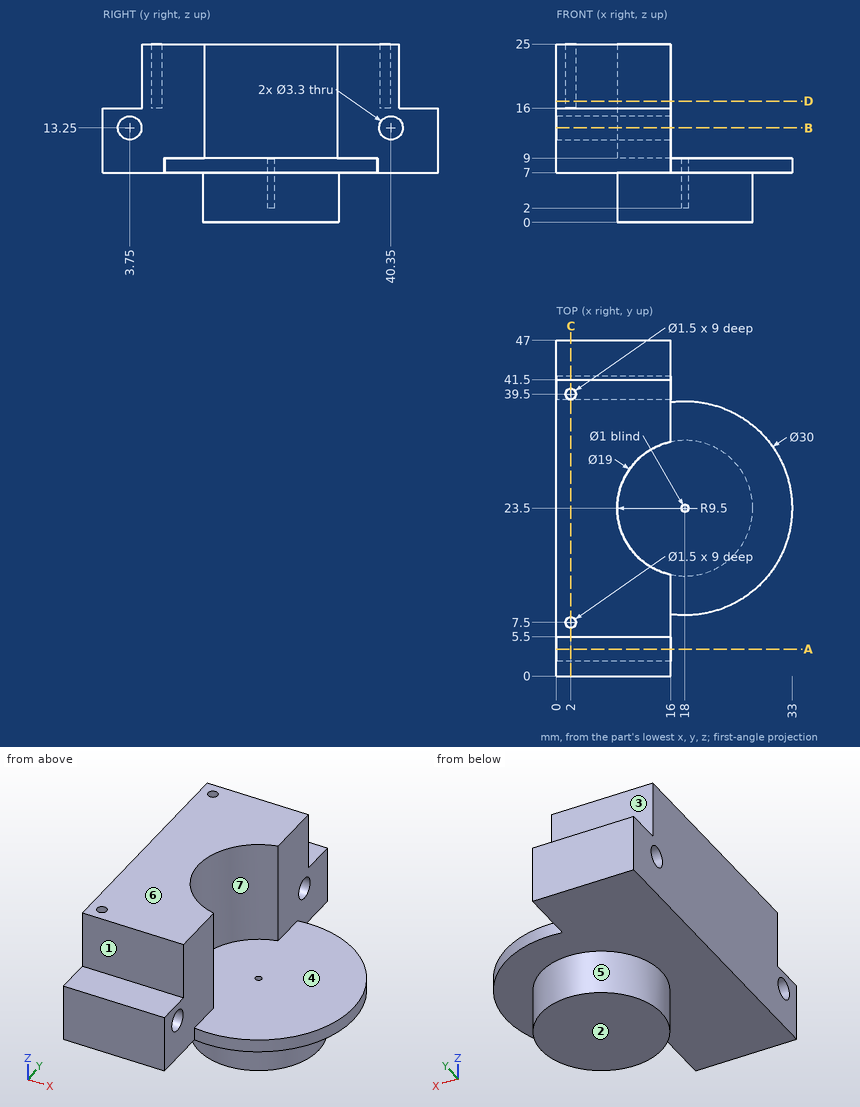
Part print with two shaded views. Sizes in mm from the minimum x, y, z corner. A direction names the side the tool comes from. Give positions to 0.01 mm unless a question says otherwise; leave off trailing zeros. Order: outer loops, then holes, each group sorted by start corner. A loop starts at its lowest first (then second) coordinate and runs counter-clockwise, first axis right, second up. Notation, with made-up numbers: M 12,18 L 46,18 A23 ccw 46,28 Z; hole C 71,-20 d6. An arc over 180 degrees is marked long. Use one line per item in the form item = value.
1) Saw through at A-A (y = 3.75). Give the cut face in (x, z), plus the area to 3 significant figures.
Calculated:
outline = M 0,7 L 16,7 L 16,11.6 L 0,11.6 Z; M 0,14.9 L 16,14.9 L 16,16 L 0,16 Z
area = 91.2 mm2
2) Saw through at D-D (z = 17). Give the cut face in (x, y), plus the area to 3 significant figures.
Calculated:
outline = M 0,5.5 L 16,5.5 L 16,14.21 A9.5 cw 16,32.79 L 16,41.5 L 0,41.5 Z; hole C 2,7.5 d1.5; hole C 2,39.5 d1.5
area = 468 mm2
3) Saw through at C-C (x = 2). Give the cut face in (y, z).
Calculated:
outline = M 0,7 L 47,7 L 47,16 L 41.5,16 L 41.5,25 L 40.25,25 L 40.25,16 L 38.75,16 L 38.75,25 L 8.25,25 L 8.25,16 L 6.75,16 L 6.75,25 L 5.5,25 L 5.5,16 L 0,16 Z; hole C 3.75,13.25 d3.3; hole C 40.35,13.25 d3.3
4) Tool access for the marked faces 1, 2, 3 and 4: list every direction of +Z, -Z, +X, -X, +Y, -Y with a clear straight run to the whole face (end or side of a thin tool).
Calculated:
face_1 = +Z, +X, -X, -Y
face_2 = -Z, +X, -X, +Y, -Y
face_3 = +Z, +X, -X, +Y
face_4 = +Z, +X
5) Probe probe 1 along Z at (x, y) = (10, 40.5); probe 2 along Y at (x, z) = (2, 19.75); probe 3 along Z at (x, y) = (27.5, 12). List the from-to ranges inside material, lowest first.
Calculated:
probe_1 = 7 to 11.61, 14.89 to 25
probe_2 = 5.5 to 6.75, 8.25 to 38.75, 40.25 to 41.5
probe_3 = 7 to 9
6) Saw through at B-B (z = 13.25). Give the cut face in (x, y).
Calculated:
outline = M 0,0 L 16,0 L 16,2.1 L 0,2.1 Z; M 0,5.4 L 16,5.4 L 16,14.21 A9.5 cw 16,32.79 L 16,38.7 L 0,38.7 Z; M 0,42 L 16,42 L 16,47 L 0,47 Z
7) Two-plate mould, pull along Y, no slides. Class the marked faces 5, 6 and 7: released by +Y, released by -Y, zero draft, split by the parting line, or undercut.
Calculated:
face_5 = split by the parting line
face_6 = zero draft
face_7 = undercut
8) Drop flat-ended pins along their axis: pin 1 (7 mm diameter, centred on y = 9, z = 19.5, fed in from +X); pin 2 (3 mm diameter, centred on x = 29, y = 20, fed in from +Z); pin 3 (1.7 mm diameter, centred on x = 2, y = 7.5, fed in from -Z). Give the stop position or say it passes through.
Calculated:
pin_1 = 16
pin_2 = 9
pin_3 = 7
